Input: part model. Units: mm. Frame: model coordinates. Face numbers are marked on the shaded views. A direction names the side the tool comes from. Coordinates: 2 decimals unless noted, no trailing zeros. Order: outer loops, then holes, each group sorted by start corner. A loop starts at its lowest first (then second) coordinate and runs counter-clockwise, first axis right, second up. Notation, with made-up numbers: (-10.75, 40) - (28.25, 40) arc R32 cw to (28.25, 70) - close; hole circle Ø3 at (29, 0.25). An arc over 180 degrees is marked (long way). One line per question, with ' | ' between items.
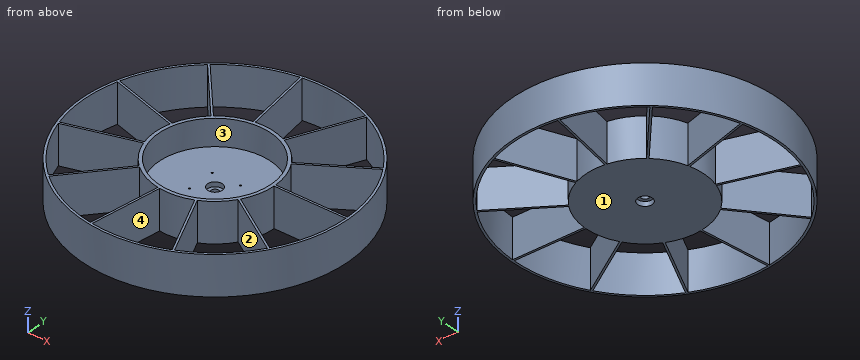
from build123d import *

# Parameters (mm, degrees)
SKETCH1_R               = 201.5
SKETCH1_R_2             = 198
RING_DEPTH              = 60
SKETCH2_R               = 90
FLOOR_2_DEPTH           = 20
SKETCH3_R               = 90
SKETCH3_R_2             = 85
HUB_TUBE_DEPTH          = 40
SKETCH4_W               = 110
SKETCH4_H               = 3
VANES_DEPTH             = 60
SKETCH5_R               = 6
BORE_DEPTH              = 20
SKETCH6_R               = 11
BEARING_SEAT_LOW_DEPTH  = 7
SKETCH7_R               = 11
BEARING_SEAT_HIGH_DEPTH = 7
SKETCH8_R               = 1.25
GROMMET_SCREWS_DEPTH    = 8


with BuildPart() as part:
    # Sketch1 → Ring (new body)
    with BuildSketch(Plane.XY):
        Circle(SKETCH1_R)
        Circle(SKETCH1_R_2, mode=Mode.SUBTRACT)
    extrude(amount=RING_DEPTH)



with BuildPart() as body_2:
    # Sketch2 → Floor 2 (new body)
    with BuildSketch(Plane.XY):
        Circle(SKETCH2_R)
    extrude(amount=FLOOR_2_DEPTH)

    # Sketch3 → Hub_tube (add)
    with BuildSketch(Plane.XY.offset(20)):
        Circle(SKETCH3_R)
        Circle(SKETCH3_R_2, mode=Mode.SUBTRACT)
    extrude(amount=HUB_TUBE_DEPTH)


with BuildPart() as part_1:
    add(part.part)

    add(body_2.part)  # Vanes merges body 2
    # Sketch4 → Vanes (add)
    with BuildSketch(Plane.XY):
        with Locations((144, 0)):
            Rectangle(SKETCH4_W, SKETCH4_H)
        Polygon((75.682525648, 46.855152454), (168.22041426, 106.325642374), (166.598491807, 108.849402973), (74.060603196, 49.378913053), align=None)
        Polygon((38.33638415, 80.334125067), (84.03203558, 180.393644556), (81.303139594, 181.639889595), (35.607488164, 81.580370106), align=None)
        Polygon((-11.181288444, 88.307580585), (-26.835920654, 197.187939192), (-29.805384979, 196.760994677), (-14.150752769, 87.88063607), align=None)
        Polygon((-57.14898096, 68.244003218), (-129.183661694, 151.376456397), (-131.450910417, 149.411874196), (-59.416229683, 66.279421017), align=None)
        Polygon((-84.972275816, 26.513437019), (-190.516502914, 57.504018272), (-191.361700585, 54.625539351), (-85.817473487, 23.634958098), align=None)
        Polygon((-85.817473487, -23.634958098), (-191.361700585, -54.625539351), (-190.516502914, -57.504018272), (-84.972275816, -26.513437019), align=None)
        Polygon((-59.416229683, -66.279421017), (-131.450910417, -149.411874196), (-129.183661694, -151.376456397), (-57.14898096, -68.244003218), align=None)
        Polygon((-14.150752769, -87.88063607), (-29.805384979, -196.760994677), (-26.835920654, -197.187939192), (-11.181288444, -88.307580585), align=None)
        Polygon((35.607488164, -81.580370106), (81.303139594, -181.639889595), (84.03203558, -180.393644556), (38.33638415, -80.334125067), align=None)
        Polygon((74.060603196, -49.378913053), (166.598491807, -108.849402973), (168.22041426, -106.325642374), (75.682525648, -46.855152454), align=None)
    extrude(amount=VANES_DEPTH)

    # Sketch5 → Bore (cut)
    with BuildSketch(Plane.XY):
        Circle(SKETCH5_R)
    extrude(amount=BORE_DEPTH, mode=Mode.SUBTRACT)

    # Sketch6 → Bearing_seat_low (cut)
    with BuildSketch(Plane.XY):
        Circle(SKETCH6_R)
    extrude(amount=BEARING_SEAT_LOW_DEPTH, mode=Mode.SUBTRACT)

    # Sketch7 → Bearing_seat_high (cut)
    with BuildSketch(Plane.XY.offset(13)):
        Circle(SKETCH7_R)
    extrude(amount=BEARING_SEAT_HIGH_DEPTH, mode=Mode.SUBTRACT)

    # Sketch8 → Grommet_screws (cut)
    with BuildSketch(Plane.XY.offset(12)):
        with Locations((21.213203436, 21.213203436)):
            Circle(SKETCH8_R)
        with Locations((-21.213203436, 21.213203436)):
            Circle(SKETCH8_R)
        with Locations((-21.213203436, -21.213203436)):
            Circle(SKETCH8_R)
        with Locations((21.213203436, -21.213203436)):
            Circle(SKETCH8_R)
    extrude(amount=GROMMET_SCREWS_DEPTH, mode=Mode.SUBTRACT)


solid = part_1.part
Item 1: Section A-A on x = 0. Return the cut outline in (y, z), and give its area (3 significant figures).
Data:
outline: (-201.5, 0) - (-198, 0) - (-198, 60) - (-201.5, 60) - close; (-90, 0) - (-11, 0) - (-11, 7) - (-6, 7) - (-6, 13) - (-11, 13) - (-11, 20) - (-85, 20) - (-85, 60) - (-90, 60) - close; (6, 7) - (11, 7) - (11, 0) - (90, 0) - (90, 60) - (85, 60) - (85, 20) - (11, 20) - (11, 13) - (6, 13) - close; (198, 0) - (201.5, 0) - (201.5, 60) - (198, 60) - close | area: 4,040 mm^2
Item 2: Section B-B on y = 157. Return the cut outline in (x, z).
Data:
outline: (-126.31, 0) - (-120.64, 0) - (-120.64, 60) - (-126.31, 60) - close; (-24.09, 0) - (-21.06, 0) - (-21.06, 60) - (-24.09, 60) - close; (70.05, 0) - (73.35, 0) - (73.35, 60) - (70.05, 60) - close; (120.64, 0) - (126.31, 0) - (126.31, 60) - (120.64, 60) - close
Item 3: Contact query for flat-ended pins moving along their axis: P1, Ø2, axis at x = 21.21, y = -21.21, coming from the +Z side; P2, Ø2, axis at x = -21, y = 21, coming from the +Z side; P3, Ø6, axis at x = 110.5, z = 15.5, coming from the +Y side. Output: stop coordinate, or through.
Data:
P1: z = 12 | P2: z = 20 | P3: y = 170.43
Item 4: Ray query, line 1 (Y direction, x = 0, z = 18); line 2 (X direction, y = -1, z = 10); line 3 (Y direction, x = 0, z = 10.3). Return the intervals inside material, ascending.
Data:
line 1: -201.5 to -198, -90 to -11, 11 to 90, 198 to 201.5 | line 2: -201.5 to -198, -89.99 to -5.92, 5.92 to 201.5 | line 3: -201.5 to -198, -90 to -6, 6 to 90, 198 to 201.5
Item 5: Section D-D on x = 105.5. Return the cut outline in (y, z), and give its area (3 significant figures).
Data:
outline: (-171.67, 0) - (-167.55, 0) - (-167.55, 60) - (-171.67, 60) - close; (-69.58, 0) - (-66.02, 0) - (-66.02, 60) - (-69.58, 60) - close; (-1.5, 0) - (1.5, 0) - (1.5, 60) - (-1.5, 60) - close; (66.02, 0) - (69.58, 0) - (69.58, 60) - (66.02, 60) - close; (167.55, 0) - (171.67, 0) - (171.67, 60) - (167.55, 60) - close | area: 1,100 mm^2
Item 6: Access query for the marked faces 3 and 4. Directions: +Z, -Z, +X, -X, +Y, -Y. A direction counts if a zero-diameter tool reaches every point of the face in a straight line with its end or side. Return the directions, or none.
Data:
face 3: +Z | face 4: +Z, -Z
Item 7: Draft query along X for the marked faces 1 and 2. Return one class per face: released by +X, released by -X, zero draft, split by the parting line, or undercut.
Data:
face 1: zero draft | face 2: undercut
Item 8: Section C-C on y = -134. Return the cut outline in (x, z), and give its area (3 significant figures).
Data:
outline: (-150.49, 0) - (-145.77, 0) - (-145.77, 60) - (-150.49, 60) - close; (-118.1, 0) - (-114.13, 0) - (-114.13, 60) - (-118.1, 60) - close; (-20.78, 0) - (-17.75, 0) - (-17.75, 60) - (-20.78, 60) - close; (59.55, 0) - (62.84, 0) - (62.84, 60) - (59.55, 60) - close; (145.77, 0) - (150.49, 0) - (150.49, 60) - (145.77, 60) - close | area: 1,180 mm^2
